```python
from build123d import *

# Parameters (mm, degrees)
F0_R     = 54.3589736978
F1_DEPTH = 121.412
F2_T     = -12.7


# Not quite as in the source:
# - a fillet or chamfer that OpenCascade refuses, or shapes differently, is made with other operations: its cross-section is extruded or revolved along the edge and cut away or added


with BuildPart() as f1:
    # F0 (on Top) → F1 (new body)
    with BuildSketch(Plane.XY):
        Circle(F0_R)
    extrude(amount=F1_DEPTH)

    # F2
    f2_openings = [f1.faces().sort_by_distance(p)[0] for p in [
        (0, 0, 121.412),
    ]]
    offset(amount=F2_T, openings=f2_openings)

    # F3: fillet of radius 15.3302561211 on 1 edges, made by hand

    # F3_s1 → F3_t2 (revolve, cut)
    with BuildSketch(Plane.XZ):
        with BuildLine():
            ThreePointArc((54.3589736978, 106.3090696395), (50.7619876396, 116.1755343746), (41.6589736978, 121.412))
            Line((41.6589736978, 121.412), (54.3589736978, 121.412))
            Line((54.3589736978, 121.412), (54.3589736978, 106.3090696395))
        make_face()
    revolve(axis=Axis((0, 0, 121.412), (0, 0, 1)), mode=Mode.SUBTRACT)


solid = f1.part
```
Part model, mm, in its own coordinate system. Coordinates: 2 decimals unless noted, no trailing zeros. Write each loop counter-clockwise with the first axis right and the second up, starting at its lowest first coordinate (ties: lowest second). Pieces come first, ordered by that corner, then holes.
Item 1: Slice it at C-C (z = 93.5). Write the cut outline in (x, y).
Item 2: Probe line 1 (Y direction, x = 0, z = 50.5); line 2 (Y direction, x = -10, z = 67); line 3 (Z direction, x = 8.5, y = -32.5). List the from-to ranges inside material, lowest first.
Item 3: Mould opens along Y. For faces 1 (the face through (-30.7, 28.16, 66.3)), 2 (the face through (-1, 1, 0)), 3 (the face through (-1, 1, 12.7)), 4 (the face through (-43.137, -33.077, 52.41)) say: released by +Y, released by -Y, zero draft, split by the parting line, or undercut.
Item 4: Slice it at A-A (x = 0). Write the cut outline in (y, z).
Item 5: Pin check, flat tips, straight feed: pin 1 (1 mm diameter, centred on y = 9.5, z = 19, fed in from +X); pin 2 (12 mm diameter, centred on y = -37.5, z = 32.5, fed in from +X); pin 3 (4 mm diameter, centred on y = -26.5, z = 41.5, fed in from -X). Stop position of each tip, or through.
Results found:
1. outline: circle Ø108.72 at (0, 0); hole circle Ø83.32 at (0, 0)
2. line 1: y = -54.36 to -41.66, 41.66 to 54.36
2. line 2: y = -53.43 to -40.44, 40.44 to 53.43
2. line 3: z = 0 to 12.7
3. face 1: undercut
3. face 2: zero draft
3. face 3: undercut
3. face 4: split by the parting line
4. outline: (-54.36, 0) - (54.36, 0) - (54.36, 106.31) arc R15.33 ccw to (41.66, 121.41) - (41.66, 12.7) - (-41.66, 12.7) - (-41.66, 121.41) arc R15.33 ccw to (-54.36, 106.31) - close
5. pin 1: stops at x = 53.61
5. pin 2: stops at x = 44.3
5. pin 3: stops at x = -48.52
